Source: CAD feature listing. Evaluate the final solid. Frame: model axes, mm. A direction names the side the tool comes from. Give positions to 0.01 mm unless a question says otherwise; leave off trailing zeros. Order: outer loops, then holes, each group sorted by start corner. A loop starts at its lowest first (then second) coordinate and runs counter-clockwise, first axis right, second up. Notation, with made-up numbers: M 40,-15 L 94,-15 A27 cw 94,15 Z; hole C -40,7.5 d11. An arc over 180 degrees is marked long. Answer in a Markdown table with one row per item. Add a question column.
(1) Section query C-C, the plane z = 5. Return loops of the section in (x, y).
(2) Section query B-B, the plane y = 0. Return loops of the section in (x, z).
(3) Mould query, pull axis Z, two halves, no side actions, for faces 1 (the face through (-9, 0, 6)), 2 (the face through (-2, 0, 0)), 3 (the face through (-10, 0, 6)), 4 (the face through (-9.507, 0.052, 5.397)). Classes: pulls with the +Z half, pulls with the -Z half, needs draft (parallel to the pull), parting line crosses it, or undercut.
(4) Section query A-A, the plane x = 0. Return loops of the section in (y, z), plus the area to 3 significant figures.
(5) Section query D-D, the plane x = -3.5. Return loops of the section in (y, z), plus the area to 3 significant figures.
(6) Pin query (flat end, axial travel): P1, Ø1, axis at y = 4, z = 3.5, coming from the +X side; P2, Ø3, axis at x = -5.5, z = 6.5, coming from the -Y side. Return the tip coordinate at first contact, or that it passes through.
(7) Material intervals for line 1 along Y through (x, z) = (0, 0.75); line 2 along Z through (x, y) = (-6.25, 4.75); line 3 along X through (y, z) = (0, 0.55), sorted ascending.
(8) Set-up query: faces 5 (the face through (-2, 0, 1)), 6 (the face through (5.498, -0.154, 0.493)), 7 (the face through (-2, 0, 10)), 8 (the face through (-9.3, -5, 5.3)), 9 (the face through (-9.3, 5, 5.3)). Return all of +Z, -Z, +X, -X, +Y, -Y with unobstructed straight access to the full face (end or side cutting, diameter ignored); none if empty.
from build123d import *

# Parameters (mm, degrees)
SKETCH1_R           = 0.4
BOSS_EXTRUDE1_DEPTH = 10
SKETCH2_W           = 8
SKETCH2_H           = 15
CUT_EXTRUDE2_DEPTH  = 19
SKETCH3_W           = 10
SKETCH3_H           = 10
BOSS_EXTRUDE2_DEPTH = 1
SKETCH4_R           = 0.4
CUT_EXTRUDE3_DEPTH  = 2


with BuildPart() as part:
    # Sketch1 → Boss-Extrude1 (new body)
    with BuildSketch(Plane.XY):
        with BuildLine():
            Line((-10, 5), (-10, -5))
            Line((-10, -5), (-2.291287847, -5))
            ThreePointArc((-2.291287847, -5), (5.5, 0), (-2.291287847, 5))
            Line((-2.291287847, 5), (-10, 5))
        make_face()
        Circle(SKETCH1_R, mode=Mode.SUBTRACT)
    extrude(amount=BOSS_EXTRUDE1_DEPTH)

    # Sketch2 → Cut-Extrude2 (cut)
    with BuildSketch(Plane.ZY.offset(10)):
        with Locations((5, 0)):
            Rectangle(SKETCH2_W, SKETCH2_H)
    extrude(amount=-CUT_EXTRUDE2_DEPTH, mode=Mode.SUBTRACT)


with BuildPart() as cut_extrude2_piece_1:
    # of the separate pieces the step leaves, piece 1, a body of its own (cut_extrude2_pieces)
    add(part.part.solids().sort_by_distance((-2.291287847, 5, 0))[0])



with BuildPart() as cut_extrude2_piece_2:
    # of the separate pieces the step leaves, piece 2, a body of its own (cut_extrude2_pieces)
    add(part.part.solids().sort_by_distance((-10, 5, 9))[0])


with BuildPart() as cut_extrude2_piece_1_1:
    add(cut_extrude2_piece_1.part)

    add(cut_extrude2_piece_2.part)  # Boss-Extrude2 merges Cut-Extrude2 piece 2
    # Sketch3 → Boss-Extrude2 (add)
    with BuildSketch(Plane.ZY.offset(10)):
        with Locations((5, 0)):
            Rectangle(SKETCH3_W, SKETCH3_H)
    extrude(amount=-BOSS_EXTRUDE2_DEPTH)

    # Sketch4 → Cut-Extrude3 (cut)
    with BuildSketch(Plane.ZY.offset(10)):
        with Locations(Location((5, 0, 0), (0, 0, 270))):
            Circle(SKETCH4_R)
    extrude(amount=-CUT_EXTRUDE3_DEPTH, mode=Mode.SUBTRACT)


solid = cut_extrude2_piece_1_1.part
Values follow:
| question | item | result |
|---|---|---|
| 1 | outline | M -10,-5 L -9,-5 L -9,-0.4 L -10,-0.4 Z; M -10,0.4 L -9,0.4 L -9,5 L -10,5 Z |
| 2 | outline | M -10,0 L -0.4,0 L -0.4,1 L -9,1 L -9,4.6 L -10,4.6 Z; M -10,5.4 L -9,5.4 L -9,9 L -0.4,9 L -0.4,10 L -10,10 Z; M 0.4,0 L 5.5,0 L 5.5,1 L 0.4,1 Z; M 0.4,9 L 5.5,9 L 5.5,10 L 0.4,10 Z |
| 3 | face 1 | undercut |
| 3 | face 2 | pulls with the -Z half |
| 3 | face 3 | needs draft |
| 3 | face 4 | undercut |
| 4 | outline | M -5.5,0 L -0.4,0 L -0.4,1 L -5.5,1 Z; M -5.5,9 L -0.4,9 L -0.4,10 L -5.5,10 Z; M 0.4,0 L 5.5,0 L 5.5,1 L 0.4,1 Z; M 0.4,9 L 5.5,9 L 5.5,10 L 0.4,10 Z |
| 4 | area | 20.4 mm² |
| 5 | outline | M -5,0 L 5,0 L 5,1 L -5,1 Z; M -5,9 L 5,9 L 5,10 L -5,10 Z |
| 5 | area | 20.0 mm² |
| 6 | P1 | stops at x = -9 |
| 6 | P2 | passes through |
| 7 | line 1 | y = -5.5 to -0.4, 0.4 to 5.5 |
| 7 | line 2 | z = 0 to 1, 9 to 10 |
| 7 | line 3 | x = -10 to -0.4, 0.4 to 5.5 |
| 8 | face 5 | +X, +Y, -Y |
| 8 | face 6 | +Z, -Z |
| 8 | face 7 | +Z, +X, -X, +Y, -Y |
| 8 | face 8 | +Z, -Z, -X, -Y |
| 8 | face 9 | +Z, -Z, -X, +Y |
